Read the model definition and answer for the solid it produces. Units are mm, in the model's axes. Face numbers are marked on the shaded views. A direction names the side the tool comes from. Coordinates: 2 decimals unless noted, no trailing zeros. Loops run counter-clockwise (first coordinate to the right, second up) from the corner with the lowest first, then second, coordinate; pieces in that order, holes last. Notation, with made-up numbers: (43, 53) - (53, 53) arc R26 cw to (53, 72) - close; hole circle Ø9 at (23.25, -30). An arc over 180 degrees is marked (long way). Use CSV: the item, a comma, the result in double quotes.
```python
from build123d import *

# Parameters (mm, degrees)
F0_R     = 12.7
F0_R_2   = 10.795
F1_DEPTH = 1.27
F0_R_3   = 7.62
F0_R_4   = 3.9751
F2_DEPTH = 19.812
F3_R     = 12.7
F3_R_2   = 10.795
F4_DEPTH = 1.27
F5_DEPTH = 6.35


with BuildPart() as f1:
    # F0 (on Top) → F1 (new body)
    with BuildSketch(Plane.XY):
        Circle(F0_R)
        Circle(F0_R_2, mode=Mode.SUBTRACT)
    extrude(amount=F1_DEPTH)

    # F0 (on Top) → F2 (join)
    with BuildSketch(Plane.XY):
        Circle(F0_R_2)
        Circle(F0_R_3, mode=Mode.SUBTRACT)
        Circle(F0_R_3)
        Circle(F0_R_4, mode=Mode.SUBTRACT)
    extrude(amount=F2_DEPTH)

    # F3 (on face) → F4 (join)
    with BuildSketch(Plane.XY.offset(19.812)):
        Circle(F3_R)
        Circle(F3_R_2, mode=Mode.SUBTRACT)
    extrude(amount=-F4_DEPTH)

    # F0 (on Top) → F5 (join)
    with BuildSketch(Plane.XY):
        Circle(F0_R_3)
        Circle(F0_R_4, mode=Mode.SUBTRACT)
    extrude(amount=-F5_DEPTH)


solid = f1.part
```
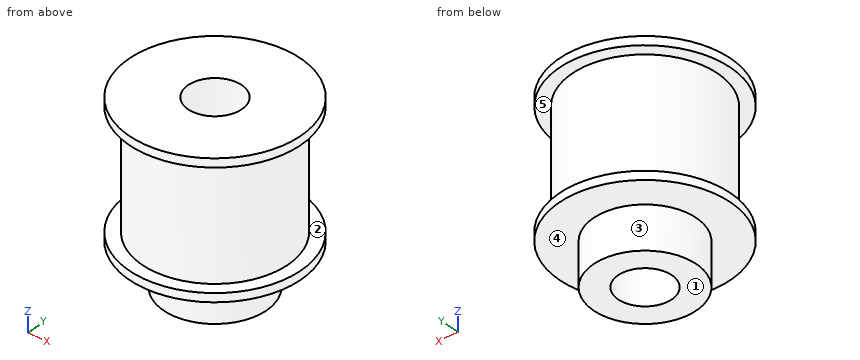
Q1. The part is cut by section C-C on z = 6.75. Determine the outline of the cut face in (x, y) (3 decimals).
Reported:
outline,"circle Ø21.59 at (0, 0); hole circle Ø7.95 at (0, 0)"
Q2. The part is cut by section D-D on y = -5.5. Determine the outline of the cut face in (x, z).
Reported:
outline,"(-11.45, 0) - (-5.27, 0) - (-5.27, -6.35) - (5.27, -6.35) - (5.27, 0) - (11.45, 0) - (11.45, 1.27) - (9.29, 1.27) - (9.29, 18.54) - (11.45, 18.54) - (11.45, 19.81) - (-11.45, 19.81) - (-11.45, 18.54) - (-9.29, 18.54) - (-9.29, 1.27) - (-11.45, 1.27) - close"
Q3. The part is cut by section A-A on x = 0. Determine the outline of the cut face in (y, z) (3 decimals).
Reported:
outline,"(-12.7, 0) - (-7.62, 0) - (-7.62, -6.35) - (-3.975, -6.35) - (-3.975, 19.812) - (-12.7, 19.812) - (-12.7, 18.542) - (-10.795, 18.542) - (-10.795, 1.27) - (-12.7, 1.27) - close; (3.975, -6.35) - (7.62, -6.35) - (7.62, 0) - (12.7, 0) - (12.7, 1.27) - (10.795, 1.27) - (10.795, 18.542) - (12.7, 18.542) - (12.7, 19.812) - (3.975, 19.812) - close"
Q4. A tool of negligible diameter and unlimited length cuts with its end or side. For the marked faces 1 and 2, from which of +Z, -Z, +X, -X, +Y, -Y can it reach the whole face along a straight path? Write none if from no direction.
Reported:
face 1,"-Z, +X, -X, +Y, -Y"
face 2,"none"
Q5. Given P1, Ø4, axis at x = 4, z = 13, coming from the +Y side; P2, Ø8, axis at x = 9.5, y = 4, coming from the -Z side; P3, Ø1, axis at x = -2.5, z = 0, coming from the -Y side; P4, Ø3, axis at x = 10, y = -5.5, coming from the -Z side, each flat-ended and moving along its own axis, determine where each tip first touches the part or whether it passes through.
Reported:
P1,"stops at y = 10.61"
P2,"stops at z = -6.35"
P3,"stops at y = -12.54"
P4,"stops at z = 0"
Q6. Find the intervals of material crossed by probe 1 along Z at (x, y) = (-4.5, -10); probe 2 along Y at (x, z) = (0, 6.5) (3 decimals); probe 3 along Z at (x, y) = (6.75, 8), in increasing order. Write a range as [from, to].
Reported:
probe 1,"z = [0, 1.27], [18.54, 19.81]"
probe 2,"y = [-10.795, -3.975], [3.975, 10.795]"
probe 3,"z = [0, 19.81]"
Q7. For a pull along Z with two mould halves and no side action, classify the marked faces 3, 4 and 5 as +Z half, -Z half, draft (parallel to the pull), parting line (faces both ways), or undercut.
Reported:
face 3,"draft"
face 4,"-Z half"
face 5,"undercut"
